Geometry check sheet. Reference: the model listing, model coordinates, mm. A direction names the side the tool comes from. Coordinates: 2 decimals unless noted, no trailing zeros. Write each loop counter-clockwise with the first axis right and the second up, starting at its lowest first coordinate (ties: lowest second). Pieces come first, ordered by that corner, then holes. Notation, with made-up numbers: (71, 45) -> (121, 45) arc R26 ccw to (121, 81) -> close; hole circle Ø3 at (-30.75, 11). An arc over 180 degrees is marked (long way). Answer in a Markdown table with one row per item. Add a question column.
1. Cross-section at B-B on x = 396. Record the cut outline in (y, z), and give its area (3 significant figures).
2. Cross-section at D-D on y = 26. Record the cut outline in (x, z).
3. Depth check by flat-ended pin: P1, Ø12, axis at y = 174, z = 296.5, coming from the -X side; P2, Ø1, axis at y = 192.5, z = 301.5, coming from the +X side; P3, Ø8, axis at x = 367.5, y = 38.5, coming from the +Z side. Enter the tip coordinate at first touch or a pass-through.
4. Cross-section at A-A on z = 129. Record the cut outline in (x, y).
5. Set-up check for faces 1 (the cylindrical face through (6.98, 5.7, 297.83)), 2 (the flat face through (152, 126, 286)), 3 (the cylindrical face through (219.705, 125.715, 270.964)): record each of +Z, -Z, +X, -X, +Y, -Y from which the full face is reachable in a straight line by a thin tool's end or side.
6. Mould release check, pull along Z, two halves, no side actions. Record for faces 4 (the flat face through (233.963, 126, 156)), 5 (the flat face through (123, 126, 0)), 6 (the flat face through (289, 215, 228)), 7 (the cylindrical face through (73.15, 68.01, 153.17)): pulls with the +Z half, pulls with the -Z half, needs draft (parallel to the pull), parting line crosses it, or undercut.
7. Cross-section at C-C on y = 127.5. Record the cut outline in (x, z), and give its area (3 significant figures).
8. Scan lines: L1, parallel to Y at x = 304, z = 335.5; L2, parallel to Z at x = 187.5, y = 161; L3, parallel to X at y = 90, z = 164. Record each from-to range of solid material in increasing order. Write a range as from..to.
Solid Edge part; units mm, degrees
sketch "Sketch1" plane through (0, 0, 0) normal (0, -1, 0) x (1, 0, 0)
  line L0 (268.9626, 310) -> (0.9626, 310)
  line L1 (0.9626, 310) -> (0.9626, 286)
  line L2 (0.9626, 286) -> (183.9626, 286)
  arc A0 (183.9626, 286) -> (233.9626, 236) centre (183.9626, 236) cw
  line L3 (233.9626, 236) -> (233.9626, 74)
  arc A1 (233.9626, 74) -> (183.9626, 24) centre (183.9626, 74) cw
  line L4 (183.9626, 24) -> (0, 24)
  line L5 (0, 24) -> (0, 0)
  line L6 (0, 0) -> (268.9626, 0)
  line L7 (268.9626, 310) -> (268.9626, 0)
extrude "Protrusion1" add sketch "Sketch1" against normal blind 255
sketch "Sketch2" plane through (134.4813, 0, 155) normal (0, -1, 0) x (1, 0, 0)
  arc A0 (216.4946, 107.8308) -> (279.1898, 72.9524) centre (279.8626, 147.9493) ccw
  arc A1 (279.1898, 72.9524) -> (309.0616, -45.7514) centre (278.6223, 9.6991) cw
  line L0 (244.7859, -73.0877) -> (309.0616, -45.7514)
  line L1 (244.7859, -73.0877) -> (134.4813, -120)
  line L2 (134.4813, -120) -> (134.4813, 155)
  line L3 (134.4813, 155) -> (-65.5187, 155)
  line L4 (-65.5187, 155) -> (-3.6234, 269.4515)
  arc A2 (40.3572, 295.6669) -> (-3.6234, 269.4515) centre (40.3572, 245.6669) ccw
  line L5 (40.3572, 295.6669) -> (64.5539, 295.6669)
  arc A3 (64.5539, 295.6669) -> (114.8016, 268.4565) centre (49.0379, 207.0144) cw
  line L6 (114.8016, 268.4565) -> (216.4946, 107.8308)
extrude "ExtrudedProtrusion_2" add sketch "Sketch2" against normal blind 40
mirror "Mirror1" about plane through (238.1797, 127.5, 225.3334) normal (0, -1, 0) of "ExtrudedProtrusion_2"
fillet "Round_1" radius 20 4 edges at (0.9626, 0, 298) (0, 0, 12) (0, 255, 12) (0.9626, 255, 298)
sketch "Sketch3" plane through (248.1797, 0, 225.3334) normal (0, -1, 0) x (1, 0, 0)
  circle A0 centre (-73.3412, 175.3334) radius 30
  circle A1 centre (164.9239, -60.6344) radius 30
extrude "Cutout1" cut sketch "Sketch3" against normal through all
sketch "Sketch4" plane through (91.9813, 117.5, 24) normal (0, 0, 1) x (1, 0, 0)
  circle A0 centre (-11.0187, 10) radius 60
  dimension "D1" = 11.0187
  dimension "D2" = 11.0187
extrude "Protrusion3" add sketch "Sketch4" along normal up to next
fillet "Round_2" radius 20 1 edges at (268.9626, 127.5, 0)
Results found:
| question | item | result |
|---|---|---|
| 1 | outline | (0, 89.03) -> (40, 89.03) -> (40, 140.05) -> (0, 140.05) -> close; (0, 189.35) -> (40, 189.35) -> (40, 230.23) -> (0, 230.23) -> close; (215, 89.03) -> (255, 89.03) -> (255, 140.05) -> (215, 140.05) -> close; (215, 189.35) -> (255, 189.35) -> (255, 230.23) -> (215, 230.23) -> close |
| 1 | area | 7,350 mm^2 |
| 2 | outline | (0, 0) -> (248.96, 0) arc R20 ccw to (268.96, 20) -> (268.96, 35) -> (379.27, 81.91) -> (443.54, 109.25) arc R63.26 ccw to (413.67, 227.95) arc R75 cw to (350.98, 262.83) -> (249.28, 423.46) arc R90 ccw to (199.04, 450.67) -> (174.84, 450.67) arc R50 ccw to (130.86, 424.45) -> (68.96, 310) -> (0.96, 310) -> (0.96, 286) -> (183.96, 286) arc R50 cw to (233.96, 236) -> (233.96, 74) arc R50 cw to (183.96, 24) -> (0, 24) -> close; hole circle Ø60 at (174.84, 400.67); hole circle Ø60 at (413.1, 164.7) |
| 3 | P1 | stops at x = 0.96 |
| 3 | P2 | stops at x = 268.96 |
| 3 | P3 | stops at z = 247.81 |
| 4 | outline | circle Ø120 at (80.96, 127.5); (233.96, 0) -> (465.32, 0) -> (465.32, 40) -> (268.96, 40) -> (268.96, 215) -> (465.32, 215) -> (465.32, 255) -> (233.96, 255) -> close |
| 5 | face 1 | +Z, -X, -Y |
| 5 | face 2 | none |
| 5 | face 3 | +Y, -Y |
| 6 | face 4 | undercut |
| 6 | face 5 | pulls with the -Z half |
| 6 | face 6 | needs draft |
| 6 | face 7 | undercut |
| 7 | outline | (0, 0) -> (248.96, 0) arc R20 ccw to (268.96, 20) -> (268.96, 310) -> (0.96, 310) -> (0.96, 286) -> (20.96, 286) -> (20.96, 24) -> (0, 24) -> close; hole (140.96, 24) -> (183.96, 24) arc R50 ccw to (233.96, 74) -> (233.96, 236) arc R50 ccw to (183.96, 286) -> (140.96, 286) -> close |
| 7 | area | 54,500 mm^2 |
| 8 | L1 | y = 0..40, 215..255 |
| 8 | L2 | z = 0..24.13, 285.87..310 |
| 8 | L3 | x = 34.13..127.8, 233.96..268.96 |
